Autodesk Inventor part; units mm, degrees
ref_plane "YZ Plane" through (0, 0, 0) normal (1, 0, 0) x (0, 1, 0)
ref_plane "XZ Plane" through (0, 0, 0) normal (0, 1, 0) x (-1, 0, 0)
ref_plane "XY Plane" through (0, 0, 0) normal (0, 0, 1) x (1, 0, 0)
sketch "Boceto1" plane through (0, 0, 0) normal (0, 1, 0) x (-1, 0, 0)
  line L0 (-1.5, -48.5) -> (1.5, -48.5)
  line L1 (1.5, -48.5) -> (1.5, 48.5)
  line L2 (1.5, 48.5) -> (-1.5, 48.5)
  line L3 (-1.5, 48.5) -> (-1.5, -48.5)
  line L4 (-1.5, -48.5) -> (1.5, 48.5) construction
  line L5 (1.5, -48.5) -> (-1.5, 48.5) construction
  point P0 (0, 0)
  dimension "d0" = 3
  dimension "d1" = 97
extrude "Extrusión1" add sketch "Boceto1" along normal blind 180
sketch "Boceto2" plane through (-1.5, 0, -48.5) normal (-1, 0, 0) x (0, 0, 1)
  circle A0 centre (24.25, 159.25) radius 1.5
  circle A1 centre (72.75, 159.25) radius 1.5
  circle A2 centre (90.5, 84) radius 1.5
  circle A3 centre (6.5, 84) radius 1.5
  circle A4 centre (6.5, 6.5) radius 1.25
  circle A5 centre (90.5, 6.5) radius 1.25
  point P0 (48.5, 0)
extrude "Extrusión2" cut sketch "Boceto2" against normal through all
sketch "Boceto3" plane through (1.5, 0, 48.5) normal (1, 0, 0) x (0, 0, -1)
  line L0 (10.5, 26) -> (5.5, 26)
  line L1 (10.5, 44) -> (10.5, 26)
  line L2 (5.5, 44) -> (-0.0781, 44)
  line L3 (-0.0781, 26) -> (5.5, 26)
  line L4 (0, 0) -> (0, 180)
  line L5 (0, 44) -> (10.5, 44)
  line L6 (10.5, 44) -> (10.5, 26)
  line L7 (10.5, 26) -> (0, 26)
  line L8 (0, 26) -> (0, 44)
  line L9 (0, 35) -> (10.5, 35)
  line L10 (10.5, 29.75) -> (0, 29.75)
  line L11 (0, 29.75) -> (0, 40.25)
  line L12 (0, 40.25) -> (10.5, 40.25)
  line L13 (10.5, 40.25) -> (10.5, 29.75)
  line L14 (10.5, 29.75) -> (0, 40.25) construction
  line L15 (0, 29.75) -> (10.5, 40.25) construction
  point P0 (48.5, 0)
  point P1 (5.25, 35)
  point P2 (10.5, 40.25)
  point P3 (10.5, 29.75)
  dimension "d13" = 10.5
extrude "Extrusión3" cut sketch "Boceto3" against normal through all contours L10 L4 L9 L1 | L9 L4 L12 L1
sketch "Boceto4" plane through (1.5, 0, 48.5) normal (1, 0, 0) x (0, 0, -1)
  line L0 (84, 0) -> (84, 13)
  line L1 (100, 0) -> (-3, 0)
  arc A0 (84, 1.85) -> (80.3, 1.85) centre (82.15, 1.85) ccw
  line L2 (0, 0) -> (97, 0)
  line L3 (80.3, 1.85) -> (80.3, 0)
  line L4 (97, 0) -> (0, 0)
  line L5 (84, 1.85) -> (84, 0)
  point P0 (48.5, 0)
  dimension "d9" = 3.7
extrude "Extrusión4" cut sketch "Boceto4" against normal through all
sketch "Boceto5" plane through (1.5, 0, -48.5) normal (1, 0, 0) x (0, 0, -1)
  line L0 (-48.5, 0) -> (-72.5, 0)
  line L1 (-16.7, 0) -> (-97, 0)
  line L2 (-72.5, 0) -> (-72.5, 30)
  line L3 (-97, 0) -> (-16.7, 0)
  line L4 (-72.5, 30) -> (-69.5, 30)
  line L5 (-69.5, 30) -> (-69.5, 51)
  line L6 (-69.5, 51) -> (-72.5, 51)
  line L7 (-72.5, 51) -> (-72.5, 30)
  line L8 (-48.5, 0) -> (-24.5, 0)
  line L9 (-24.5, 0) -> (-24.5, 30)
  line L10 (-24.5, 30) -> (-27.5, 30)
  line L11 (-27.5, 30) -> (-27.5, 51.0089)
  line L12 (-27.5, 51.0089) -> (-24.5, 51.0089)
  line L13 (-24.5, 51.0089) -> (-24.5, 30)
  line L14 (-72.5, 51) -> (-72.5, 101)
  line L15 (-72.5, 101) -> (-69.5, 101)
  line L16 (-69.5, 101) -> (-69.5, 122)
  line L17 (-69.5, 122) -> (-72.5, 122)
  line L18 (-72.5, 122) -> (-72.5, 101)
  line L19 (-27.5, 101) -> (-24.5, 101)
  line L20 (-24.5, 101) -> (-24.5, 122)
  line L21 (-24.5, 122) -> (-27.5, 122)
  line L22 (-27.5, 122) -> (-27.5, 101)
  dimension "d14" = 24
  dimension "d15" = 30
  dimension "d16" = 3
  dimension "d17" = 21
  dimension "d18" = 24
  dimension "d19" = 30
  dimension "d20" = 3
  dimension "d21" = 50
  dimension "d22" = 21
extrude "Extrusión5" cut sketch "Boceto5" against normal blind 10
properties part number "Panel2"
Input: part model. Units: mm. Frame: model coordinates. Coordinates: 2 decimals unless noted, no trailing zeros. Loops run counter-clockwise (first coordinate to the right, second up) from the corner with the lowest first, then second, coordinate; pieces in that order, holes last.
Q1. Cut plane A-A (y = 36.5). Output: boundary loops of the cut face in (x, z), then the cut area to 4 significant figures.
Q2. Material intervals for line 1 (Y direction, x = -0.35, z = -42); line 2 (Z direction, x = -0.35, y = 159.25); line 3 (Z direction, x = -0.2, y = 119.5), sorted ascending.
Q3. Contact query for flat-ended pins moving along their axis: pin 1 (1.5 mm diameter, centred on x = 0, z = -22.5, fed in from -Y); pin 2 (0.9 mm diameter, centred on x = 0, y = 39.5, fed in from +Z). Output: stop coordinate, or through.
Q4. Cut plane B-B (x = 0.5). Give the number of separate pieces and of enclosed holes in the cut face, then the cut area to 3 significant figures.
Working result:
1. outline: (-1.5, -48.5) - (1.5, -48.5) - (1.5, -24) - (-1.5, -24) - close; (-1.5, -21) - (1.5, -21) - (1.5, 21) - (-1.5, 21) - close; (-1.5, 24) - (1.5, 24) - (1.5, 38) - (-1.5, 38) - close
1. area: 241.5 mm2
2. line 1: y = 0 to 5.25, 7.75 to 82.5, 85.5 to 180
2. line 2: z = -48.5 to -25.75, -22.75 to 22.75, 25.75 to 48.5
2. line 3: z = -48.5 to -24, -21 to 21, 24 to 48.5
3. pin 1: stops at y = 0
3. pin 2: stops at z = 38
4. separate pieces: 1
4. enclosed holes: 10
4. area: 17,000 mm2
